from build123d import *

# Parameters (mm, degrees)
SKETCH1_W           = 15
SKETCH1_H           = 10
BOSS_EXTRUDE1_DEPTH = 50
CUT_EXTRUDE1_DEPTH  = 25
SKETCH3_R           = 2
CUT_EXTRUDE2_DEPTH  = 25


with BuildPart() as part:
    # Sketch1 → Boss-Extrude1 (new body)
    with BuildSketch(Plane.XY):
        Rectangle(SKETCH1_W, SKETCH1_H)
    extrude(amount=BOSS_EXTRUDE1_DEPTH)

    # Sketch2 → Cut-Extrude1 (cut)
    with BuildSketch(Plane.XY.offset(50)):
        with BuildLine():
            Line((-3, 1), (3, 1))
            ThreePointArc((3, 1), (4, 0), (3, -1))
            Line((3, -1), (-3, -1))
            ThreePointArc((-3, -1), (-4, 0), (-3, 1))
        make_face()
    extrude(amount=-CUT_EXTRUDE1_DEPTH, mode=Mode.SUBTRACT)

    # Sketch3 → Cut-Extrude2 (cut)
    with BuildSketch(Plane(origin=(0, 0, 0), x_dir=(-1, 0, 0), z_dir=(0, 0, -1))):
        Circle(SKETCH3_R)
    extrude(amount=-CUT_EXTRUDE2_DEPTH, mode=Mode.SUBTRACT)


solid = part.part
Verification items for the finished model (mm, model axes). A direction names the side the tool comes from. Give positions to 0.01 mm unless a question says otherwise; leave off trailing zeros. Write each loop counter-clockwise with the first axis right and the second up, starting at its lowest first coordinate (ties: lowest second). Pieces come first, ordered by that corner, then holes. Notation, with made-up numbers: M -31,-23.5 L 6,-23.5 A27 ccw 6,14.5 Z; hole C 77,77 d5. An arc over 180 degrees is marked long. Write item = value, one per line.
(1) Sectioned sample at C-C (y = 0.5). Record the cut outline in (x, z).
Found:
outline = M -7.5,0 L -1.94,0 L -1.94,25 L -3.87,25 L -3.87,50 L -7.5,50 Z; M 1.94,0 L 7.5,0 L 7.5,50 L 3.87,50 L 3.87,25 L 1.94,25 Z
(2) Go/stop test with a flat-tipped pin: pin 1 Ø2 at (x, y) = (-3, -0.5) entering from +Z. Record where the tip stops, or that it passes through.
Found:
pin_1 = 50
(3) Access from +Z, -Z, +X, -X, +Y, -Y to the whole of each face (thin tool, end or side, straight path). Record for faces 4 (the face through (0, -1, 38)), 5 (the face through (0, -1.4, 25)), 6 (the face through (0, -5, 25)).
Found:
face_4 = +Z
face_5 = -Z
face_6 = +Z, -Z, +X, -X, -Y
(4) Draft check along Y on faces 1 (the face through (0, 5, 25)), 2 (the face through (-2, -1, 0)), 3 (the face through (0, 1, 38)). Enter one of: released by +Y, released by -Y, zero draft, split by the parting line, or undercut.
Found:
face_1 = released by +Y
face_2 = zero draft
face_3 = undercut
(5) Sectioned sample at A-A (x = 0). Record the cut outline in (y, z), then the cut area to 3 significant figures.
Found:
outline = M -5,0 L -2,0 L -2,25 L -1,25 L -1,50 L -5,50 Z; M 1,25 L 2,25 L 2,0 L 5,0 L 5,50 L 1,50 Z
area = 350 mm2
(6) Sectioned sample at B-B (z = 29). Record the cut outline in (x, y).
Found:
outline = M -7.5,-5 L 7.5,-5 L 7.5,5 L -7.5,5 Z; hole M -3,-1 L 3,-1 A1 ccw 3,1 L -3,1 A1 ccw Z
(7) Sectioned sample at D-D (z = 23). Record the cut outline in (x, y), then the cut area to 3 significant figures.
Found:
outline = M -7.5,-5 L 7.5,-5 L 7.5,5 L -7.5,5 Z; hole C 0,0 d4
area = 137 mm2
(8) Material ranges on line 1 (Y direction, x = 0, z = 9.5); line 2 (Y direction, x = -1.5, z = 40); line 3 (X direction, y = 0, z = 17.5), recorded low to high.
Found:
line_1 = -5 to -2, 2 to 5
line_2 = -5 to -1, 1 to 5
line_3 = -7.5 to -2, 2 to 7.5
